Geometry check sheet. Reference: drawing and pictorial views, mm from the part's lowest x, y, z. Coordinates: 2 decimals unless noted, no trailing zeros. Loops run counter-clockwise (first coordinate to the right, second up) from the corner with the lowest first, then second, coordinate; pieces in that order, holes last. Notation, with made-up numbers: (10, -34.5) -> (52, -34.5) arc R28 ccw to (52, -3.5) -> close; hole circle Ø5 at (-17.75, 68). An arc over 180 degrees is marked (long way). Answer as a JSON object with one key per item and string values.
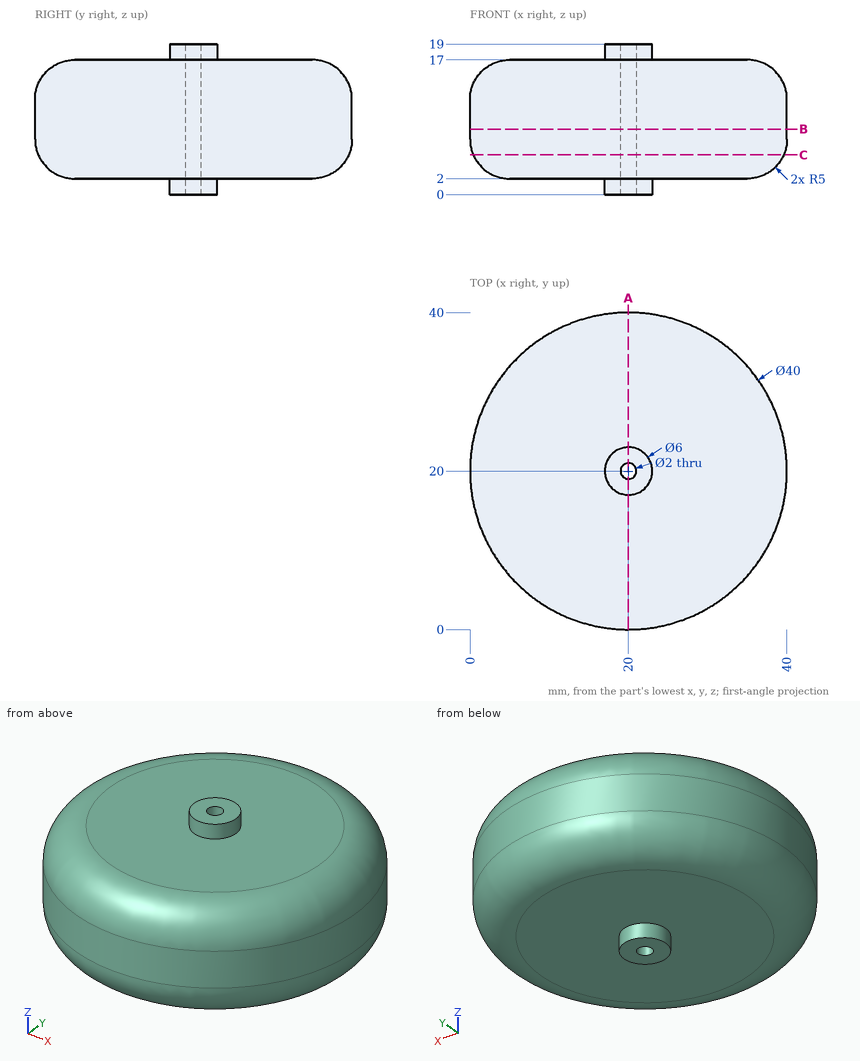
1. Section check B-B, the plane z = 8.25. Record the boundary of the cut face in (x, y).
Evaluation:
{"outline": "circle Ø40 at (20, 20); hole circle Ø2 at (20, 20)"}
2. Depth check by flat-ended pin: P1, Ø5, axis at y = 10, z = 10, coming from the -X side; P2, Ø1.5, axis at x = 35, y = 16.5, coming from the -Z side; P3, Ø5, axis at x = 9.5, z = 10, coming from the -Y side. Enter the tip coordinate at first touch or a pass-through.
Evaluation:
{"P1": "stops at x = 1.46", "P2": "stops at z = 2", "P3": "stops at y = 1.67"}
3. Thickness scan on probe 1 along Y at (x, z) = (20, 9.25); probe 2 along Z at (x, y) = (15, 17); probe 3 along X at (y, z) = (13.5, 13). Record the ranges inside material, lowest first. Write a range as from..to.
Evaluation:
{"probe 1": "y = 0..19, 21..40", "probe 2": "z = 2..17", "probe 3": "x = 1.19..38.81"}
4. Section check A-A, the plane x = 20. Record the boundary of the cut face in (y, z).
Evaluation:
{"outline": "(0, 7) arc R5 ccw to (5, 2) -> (17, 2) -> (17, 0) -> (19, 0) -> (19, 19) -> (17, 19) -> (17, 17) -> (5, 17) arc R5 ccw to (0, 12) -> close; (21, 0) -> (23, 0) -> (23, 2) -> (35, 2) arc R5 ccw to (40, 7) -> (40, 12) arc R5 ccw to (35, 17) -> (23, 17) -> (23, 19) -> (21, 19) -> close"}
5. Section check C-C, the plane z = 5. Record the boundary of the cut face in (x, y), then the cut area to 3 significant figures.
Evaluation:
{"outline": "circle Ø39.17 at (20, 20); hole circle Ø2 at (20, 20)", "area": "1,200 mm^2"}
